```python
from build123d import *

# Parameters (mm, degrees)
SKETCH_1_R               = 12.5
SKETCH_1_R_2             = 2.6
EXTRUDE_1_DEPTH          = 5
SKETCH_1_4_R             = 5
SKETCH_1_4_R_2           = 2.6
EXTRUDE_2_DEPTH          = 14
CUT_EXTRUDE_1_DEPTH      = 10
CUT_EXTRUDE_1_DEPTH_BACK = 10
SKETCH_2_R               = 1.6


with BuildPart() as part:
    # 草图1 → 凸台-拉伸1 (new body)
    with BuildSketch(Plane.XY):
        Circle(SKETCH_1_R)
        Circle(SKETCH_1_R_2, mode=Mode.SUBTRACT)
    extrude(amount=EXTRUDE_1_DEPTH)

    # 草图1<4> → 凸台-拉伸2 (add)
    with BuildSketch(Plane.XY):
        Circle(SKETCH_1_4_R)
        Circle(SKETCH_1_4_R_2, mode=Mode.SUBTRACT)
    extrude(amount=EXTRUDE_2_DEPTH)

    # 草图2 → 切除-拉伸1 (cut, two sides: drawn at the far end of the back side and taken through both)
    with BuildSketch(Plane(origin=(0, 0, 0), x_dir=(0, 0, -1), z_dir=(1, 0, 0)).offset(-CUT_EXTRUDE_1_DEPTH_BACK)):
        with Locations(Location((-11, 0, 0), (0, 0, 180))):
            Circle(SKETCH_2_R)
    extrude(amount=CUT_EXTRUDE_1_DEPTH + CUT_EXTRUDE_1_DEPTH_BACK, mode=Mode.SUBTRACT)


solid = part.part
```
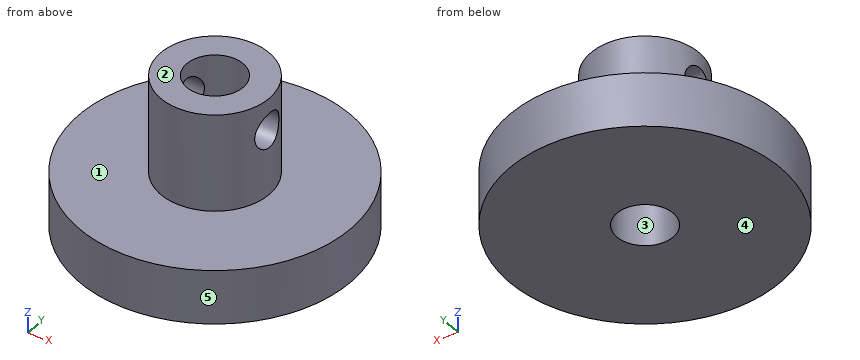
CAD build for the part. Positions are in the model's coordinates, mm. Face numbers are marked on the shaded views. A direction names the side the tool comes from. Coordinates: 2 decimals unless noted, no trailing zeros. Order: outer loops, then holes, each group sorted by start corner. A loop starts at its lowest first (then second) coordinate and runs counter-clockwise, first axis right, second up. Notation, with made-up numbers: (69.5, -24) - (108.5, -24) arc R29 cw to (108.5, 12) - close; hole circle Ø10 at (9.5, 28). An arc over 180 degrees is marked (long way). Use a Markdown table: item, result. Add a question column.
(1) Which spindle directions (+Z, -Z, +X, -X, +Y, -Y) get a long thin tool onto all of the face, cutting with end or side? Do the marked faces 1 and 2. Say none if no direction does.
(2) Pull direction X, two halves, no side cores. Call the marked faces 3, 4 and 5: +X half, -X half, draft (parallel to the pull), parting line (faces both ways), or undercut.
(3) Flat gauge pins, fed straight in: pin 1 (3 mm diameter, centred on x = 0, y = 0, fed in from -Z); pin 2 (5 mm diameter, centred on y = 0, z = 11, fed in from -X); pin 3 (6 mm diameter, centred on x = 5.5, z = 10.5, fed in from +Y); pin 4 (6 mm diameter, centred on x = 9, y = 5.5, fed in from +Z). Where does each tip first touch, or does it go through?
(4) Saw through at C-C (z = 10.25). Give the cut face in (x, y).
(5) Saw through at A-A (y = 0). Give the cut face in (x, z), then the cut area to 3 significant figures.
(6) Drill centre lines: line 1 along Y through (x, z) = (0, 6); line 2 along Z through (x, y) = (9, 6). Where is each one in solid material? Low to high. Write a range as [from, to].
(7) Saw through at D-D (z = 3.25). Give the cut face in (x, y), then the cut area to 3 significant figures.
(8) Saw through at B-B (x = 0). Give the cut face in (y, z).
Solved:
| question | item | result |
|---|---|---|
| 1 | face 1 | +Z |
| 1 | face 2 | +Z, +X, -X, +Y, -Y |
| 2 | face 3 | undercut |
| 2 | face 4 | draft |
| 2 | face 5 | parting line |
| 3 | pin 1 | passes through |
| 3 | pin 2 | stops at x = -5 |
| 3 | pin 3 | stops at y = 4.33 |
| 3 | pin 4 | stops at z = 5 |
| 4 | outline | (-4.8, -1.41) arc R5 ccw to (4.8, -1.41) - (2.18, -1.41) arc R2.6 cw to (-2.18, -1.41) - close; (-4.8, 1.41) - (-2.18, 1.41) arc R2.6 cw to (2.18, 1.41) - (4.8, 1.41) arc R5 ccw to start |
| 5 | outline | (-12.5, 0) - (-2.6, 0) - (-2.6, 9.4) - (-5, 9.4) - (-5, 5) - (-12.5, 5) - close; (-5, 12.6) - (-2.6, 12.6) - (-2.6, 14) - (-5, 14) - close; (2.6, 0) - (12.5, 0) - (12.5, 5) - (5, 5) - (5, 9.4) - (2.6, 9.4) - close; (2.6, 12.6) - (5, 12.6) - (5, 14) - (2.6, 14) - close |
| 5 | area | 127 mm² |
| 6 | line 1 | y = [-5, -2.6], [2.6, 5] |
| 6 | line 2 | z = [0, 5] |
| 7 | outline | circle Ø25 at (0, 0); hole circle Ø5.2 at (0, 0) |
| 7 | area | 470 mm² |
| 8 | outline | (-12.5, 0) - (-2.6, 0) - (-2.6, 14) - (-5, 14) - (-5, 5) - (-12.5, 5) - close; (2.6, 0) - (12.5, 0) - (12.5, 5) - (5, 5) - (5, 14) - (2.6, 14) - close |
